from build123d import *

# Parameters (mm, degrees)
F0_R     = 12.7
F1_DEPTH = 30.1625
F3_DEPTH = 19.05
F5_DEPTH = 19.05
F6_R     = 6.35
F7_DEPTH = 22.353
F8_R     = 5.08


with BuildPart() as f1:
    # F0 (on Front) → F1 (new body, symmetric)
    with BuildSketch(Plane.XZ):
        with BuildLine():
            Line((100.4062, 0), (-63.5762, 0))
            ThreePointArc((-63.5762, 0), (-101.733451, 15.805251), (-85.9282, -22.352))
            Line((-85.9282, -22.352), (108.2802, -22.352))
            Line((108.2802, -22.352), (108.2802, -7.874))
            ThreePointArc((108.2802, -7.874), (105.973959, -2.306241), (100.4062, 0))
        make_face()
        with Locations((-85.9282, 0)):
            Circle(F0_R, mode=Mode.SUBTRACT)
    extrude(amount=F1_DEPTH, both=True)

    # F2 (on face) → F3 (cut)
    with BuildSketch(Plane.XZ.offset(30.1625)):
        Polygon((31.3182, 0), (-0.0762, 0), (5.9182, -22.352), (31.3182, -22.352), align=None)
    extrude(amount=-F3_DEPTH, mode=Mode.SUBTRACT)

    # F4 (on face) → F5 (join)
    with BuildSketch(Plane.XZ.offset(30.1625)):
        with BuildLine():
            ThreePointArc((64.1604, 29.718), (62.672502, 33.310102), (59.0804, 34.798))
            Line((59.0804, 34.798), (45.1104, 34.798))
            ThreePointArc((45.1104, 34.798), (41.536215, 16.082358), (31.3182, 0))
            Line((31.3182, 0), (64.1604, 0))
            Line((64.1604, 0), (64.1604, 29.718))
        make_face()
    extrude(amount=-F5_DEPTH)

    # F6 (on face) → F7 (cut, through all)
    with BuildSketch(Plane.XY):
        with Locations((69.4182, 7.8105)):
            Circle(F6_R)
    extrude(amount=-F7_DEPTH, mode=Mode.SUBTRACT)

    # F8
    f8_edges = [f1.edges().sort_by_distance(p)[0] for p in [
        (-63.5762, 0, 0),
    ]]
    fillet(f8_edges, radius=F8_R)


solid = f1.part
Build history of the part. All positions in model axes, mm. A direction names the side the tool comes from. Coordinates: 2 decimals unless noted, no trailing zeros. Write each loop counter-clockwise with the first axis right and the second up, starting at its lowest first coordinate (ties: lowest second). Pieces come first, ordered by that corner, then holes.
(1) Mould opens along Z. For faces 1 (the cylindrical face through (-98.616, 0.422, 0.558)), 2 (the cylindrical face through (62.71, -20.77, 33.27)), 3 (the cylindrical face through (75.475, 9.718, -11.02)) say: pulls with the +Z half, pulls with the -Z half, needs draft (parallel to the pull), parting line crosses it, or undercut.
(2) Pin check, flat tips, straight feed: pin 1 Ø15 at (y, z) = (-17.5, 21) entering from +X; pin 2 Ø6.5 at (x, z) = (23, -12.5) entering from -Y; pin 3 Ø9.5 at (y, z) = (-20, -11) entering from -X; pin 4 Ø11.5 at (x, y) = (69.42, 7.81) entering from -Z (3 decimals). Stop position of each tip, or through.
(3) Cut at D-D on y = 5.5. List the corners of the cut face in (x, z), and give its area (3 significant figures).
(4) Cut at C-C on x = -84. List the corners of the cut face in (y, z).
(5) Cut at A-A on y = -20.5. List the corners of the cut face in (x, z), and give its area (3 significant figures).
(6) Cut at B-B on y = 21. List the corners of the cut face in (x, z), and give its area (3 significant figures).
(7) Drill centre lines: line 1 (Y direction, x = 11.5, z = -4.5); line 2 (Z direction, x = 10.5, y = -6); line 3 (X direction, y = 11, z = -4). Where is each one in solid material? Low to high.
(8) 3-axis set-ups, long thin cutter, end or side, ignore diameter. For faces 4 (the flat face through (31.318, -21, -11)), 5 (the flat face through (2.88, -20.77, -11.02)), 6 (the cylindrical face through (-62, 0, 1)): which of +Z, -Z, +X, -X, +Y, -Y reach the whole face in a straight line?
Working result:
1. face 1: undercut
1. face 2: pulls with the +Z half
1. face 3: needs draft
2. pin 1: stops at x = 64.16
2. pin 2: stops at y = -11.11
2. pin 3: stops at x = -107.39
2. pin 4: passes through
3. outline: (-85.93, -22.35) - (63.5, -22.35) - (63.5, 0) - (-58.97, 0) arc R5.08 cw to (-63.96, 4.14) arc R22.35 ccw (long way) to start; (75.33, -22.35) - (108.28, -22.35) - (108.28, -7.87) arc R7.87 ccw to (100.41, 0) - (75.33, 0) - close; hole circle Ø25.4 at (-85.93, 0)
3. area: 4,740 mm2
4. outline: (-30.16, -22.35) - (30.16, -22.35) - (30.16, -12.55) - (-30.16, -12.55) - close; (-30.16, 12.55) - (30.16, 12.55) - (30.16, 22.27) - (-30.16, 22.27) - close
5. outline: (-85.93, -22.35) - (5.92, -22.35) - (-0.08, 0) - (-58.97, 0) arc R5.08 cw to (-63.96, 4.14) arc R22.35 ccw (long way) to start; (31.32, -22.35) - (108.28, -22.35) - (108.28, -7.87) arc R7.87 ccw to (100.41, 0) - (64.16, 0) - (64.16, 29.72) arc R5.08 ccw to (59.08, 34.8) - (45.11, 34.8) arc R50.8 cw to (31.32, 0) - close; hole circle Ø25.4 at (-85.93, 0)
5. area: 5,170 mm2
6. outline: (-85.93, -22.35) - (108.28, -22.35) - (108.28, -7.87) arc R7.87 ccw to (100.41, 0) - (-58.97, 0) arc R5.08 cw to (-63.96, 4.14) arc R22.35 ccw (long way) to start; hole circle Ø25.4 at (-85.93, 0)
6. area: 5,000 mm2
7. line 1: y = -11.11 to 30.16
7. line 2: z = -22.35 to 0
7. line 3: x = -107.92 to -97.98, -73.87 to 63.93, 74.91 to 107.26
8. face 4: +Z, -Z, -Y
8. face 5: +Z, -Y
8. face 6: +Z, +Y, -Y
